Autodesk Fusion 360 part; units mm, degrees
sketch "ratchet" plane through (0, 0, 0) normal (0, 1, 0) x (1, 0, 0)
  circle A0 centre (0, 0) radius 6.5
  circle A1 centre (0, 0) radius 1.5
  circle A2 centre (0, 0) radius 2
  line L0 (0, 0) -> (1.3457, -7.6321)
  line L1 (0, 0) -> (-2.8494, -5.8422)
  arc A3 (-2.8494, -5.8422) -> (1.3457, -7.6321) centre (0.5378, -3.7146) ccw
  line L2 (0, 0) -> (7.7499, 0) construction
  arc A4 (1.3457, -7.6321) -> (0.8742, -7.7004) centre (0, 0) ccw
  dimension "d1" = 13
  dimension "d2" = 4
  dimension "d3" = 3
  dimension "d5" = 7.6321
  dimension "d6" = 36
  dimension "d7" = 4
  dimension "d12" = 80
extrude "Extrude1" add sketch "ratchet" against normal blind 5 contours A0 A2 L0 L1 | A0 L0 A3 picked at (-1.3488, -4.8046) makes body 1
pattern_circular "C-Pattern1" count 10 over 360 about axis through (0, -5, 0) along (0, 1, 0) of bodies 1 makes body 2 at (2.8174, -1.6667, 2.7207) makes body 3 at (3.8785, -3.3333, 0.5451) makes body 4 at (3.4582, -3.3333, -1.8387) makes body 5 at (1.7169, -1.6667, -3.5202) makes body 6 at (-0.6801, -1.6667, -3.8571) makes body 7 at (-2.8174, -3.3333, -2.7207) makes body 8 at (-3.8785, -3.3333, -0.5451) makes body 9 at (-3.4582, -1.6667, 1.8387) makes body 10 at (-1.7169, -1.6667, 3.5202)
extrude "Extrude2" add sketch "ratchet" against normal blind 5 contours A1 A2 L0 L1 | A1 A2 L0 L1 bodies 1 2 3 4 5 6 7 8 9 10
CAD build for the part. Positions are in the model's coordinates, mm. A direction names the side the tool comes from. Round coordinates to 2 decimals unless told otherwise and drop trailing zeros. Write each loop counter-clockwise with the first axis right and the second up, starting at its lowest first coordinate (ties: lowest second). Pieces come first, ordered by that corner, then holes. Notation, with made-up numbers: M 42.5,23.5 L 67.5,23.5 A18 cw 67.5,40.5 Z; hole C 37.5,-3 d1. An arc over 180 degrees is marked long. One line per question, with ' | ' between items.
1. Cut at D-D on x = 3.75. Write the cut outline in (y, z).
Working result:
outline: M -5,-6.78 L 0,-6.78 L 0,6.53 L -5,6.53 Z
2. Probe L1, parallel to Z at x = 0, y = -3.8; L2, parallel to X at y = -3.8, z = 0; L3, parallel to X at y = -4.5, z = 6 (3 decimals). List the from-to ranges inside material, lowest first. Write a range as from..to.
Working result:
L1: -7.68..-1.5, 1.5..7.68 | L2: -7.01..-1.5, 1.5..7.01 | L3: -4.719..-2.926, -2.745..4.863
3. Pin check, flat tips, straight feed: pin 1 Ø1.5 at (x, y) = (5, -3) entering from -Z; pin 2 Ø2.5 at (x, z) = (0, 0) entering from +Y; pin 3 Ø2 at (y, z) = (-2.5, 5.5) entering from +X. Stop position of each tip, or through.
Working result:
pin 1: z = -6.44 | pin 2: through | pin 3: x = 5.57
4. Which spindle directions (+Z, -Z, +X, -X, +Y, -Y) get a long thin tool onto all of the face, cutting with end or side? Do faces 4 (the flat face through (-1.236, -2.465, -7.008)), 5 (the flat face through (-7.05, -2.46, -0.99)), 6 (the flat face through (5.119, -2.465, 4.943)). Say none if no direction does.
Working result:
face 4: +Y, -Y | face 5: -X, +Y, -Y | face 6: +X, +Y, -Y
5. Mould opens along X. For faces 1 (the flat face through (-5.119, -2.465, -4.943)), 2 (the flat face through (7.05, -2.46, 0.99)), 3 (the cylindrical face through (-3.478, -2.465, -6.596)) say: pulls with the +X half, pulls with the -X half, needs draft (parallel to the pull), parting line crosses it, or undercut.
Working result:
face 1: pulls with the -X half | face 2: pulls with the +X half | face 3: undercut
6. Cut at B-B on z = 0. Write the cut outline in (x, y), and give its area (3 significant figures).
Working result:
outline: M -7.01,-5 L -1.5,-5 L -1.5,0 L -7.01,0 Z; M 1.5,-5 L 7.01,-5 L 7.01,0 L 1.5,0 Z | area: 55.1 mm2
7. Cut at A-A on y = -1.8. Write the cut outline in (x, z).
Working result:
outline: M -7.67,-1.08 A4 ccw -4.68,-4.52 L -5.57,-5.38 A4 ccw -1.13,-6.4 L -1.35,-7.63 A4 ccw 2.85,-5.84 L 3.4,-6.97 A4 ccw 5.74,-3.05 L 6.84,-3.64 A4 ccw 6.44,0.9 L 7.67,1.08 A4 ccw 4.68,4.52 L 5.57,5.38 A4 ccw 1.13,6.4 L 1.35,7.63 A4 ccw -2.85,5.84 L -3.4,6.97 A4 ccw -5.74,3.05 L -6.84,3.64 A4 ccw -6.44,-0.9 Z; hole C 0,0 d3
8. Cut at C-C on x = 0. Write the cut outline in (y, z), and give its area (3 significant figures).
Working result:
outline: M -5,-7.68 L 0,-7.68 L 0,-1.5 L -5,-1.5 Z; M -5,1.5 L 0,1.5 L 0,7.68 L -5,7.68 Z | area: 61.8 mm2
